Autodesk Inventor part; units mm, degrees
ref_plane "YZ Plane" through (0, 0, 0) normal (1, 0, 0) x (0, 1, 0)
ref_plane "XZ Plane" through (0, 0, 0) normal (0, 1, 0) x (-1, 0, 0)
ref_plane "XY Plane" through (0, 0, 0) normal (0, 0, 1) x (1, 0, 0)
sketch "スケッチ1" plane through (0, 0, 0) normal (0, 1, 0) x (-1, 0, 0)
  line L0 (0, -21.0065) -> (0, 21.0391)
  line L1 (-95.27, 0) -> (121.47, 0)
  line L2 (22, -15) -> (-22, -15)
  line L3 (-22, -15) -> (-22, 15)
  line L4 (-22, 15) -> (22, 15)
  line L5 (22, 15) -> (22, -15)
  line L6 (6, 15) -> (2.9, 15)
  line L7 (2.9, 15) -> (2.9, 11.5)
  line L8 (2.9, 11.5) -> (6, 11.5)
  line L9 (6, 11.5) -> (6, 15)
  arc A0 (10.85, 15) -> (9.45, 0) centre (90.5071, 0) ccw
  arc A1 (16.75, 0) -> (15.35, 15) centre (-64.3071, 0) ccw
  line L10 (13.1, -2.0457) -> (13.1, 1.915)
  line L11 (16.75, 0) -> (9.45, 0)
  line L12 (15.35, 15) -> (10.85, 15)
  line L13 (16.5956, 5) -> (9.6044, 5)
  line L14 (19.25, -15) -> (19.25, 15)
  point P0 (0, 0)
  point P1 (2.9, 15)
  point P2 (19.25, 0)
  point P3 (22, 0)
  dimension "d0" = 44
  dimension "d1" = 30
  dimension "d18" = 3.5
  dimension "d19" = 6
  dimension "d20" = 3.1
  dimension "d21" = 16.75
  dimension "d22" = 7.3
  dimension "d25" = 4.5
  dimension "d26" = 10
  dimension "d28" = 6.9913
  dimension "d37" = 2.9
  dimension "d38" = 19.25
extrude "押し出し1" add sketch "スケッチ1" against normal blind 2
extrude "押し出し3" add sketch "スケッチ1" along normal blind 3 contours L4 L9 L8 L7 | A0 L4 A1 L13
extrude "押し出し4" add sketch "スケッチ1" along normal blind 1.5 contours A0 L13 A1 L1
mirror "ミラー1" about plane through (0, 0, 0) normal (0, 0, 1) of "押し出し1", "押し出し3", "押し出し4"
extrude "押し出し5" add sketch "スケッチ1" along normal blind 4.2 contours L14 L1 L5 L2 | L14 L4 L5 L1
mirror "ミラー3" about plane through (0, 0, 0) normal (1, 0, 0) of "押し出し1", "押し出し3", "押し出し4", "ミラー1", "押し出し5"
sketch "スケッチ2" plane through (0, 0, 0) normal (0, 0, 1) x (1, 0, 0)
  line L0 (0, 5.44) -> (0, -3.24)
  line L1 (-30.8, 0) -> (30.8, 0)
  line L2 (-29.5, 14.3) -> (-27.5, 14.3)
  line L3 (-27.5, 14.3) -> (-27.5, 0)
  line L4 (27.5, 0) -> (27.5, 14.3)
  line L5 (27.5, 14.3) -> (29.5, 14.3)
  line L6 (29.5, 14.3) -> (29.5, -1.4)
  line L7 (29.5, -1.4) -> (25, -5.9)
  line L8 (25, -5.9) -> (-25, -5.9)
  line L9 (-25, -5.9) -> (-29.5, -1.4)
  line L10 (-29.5, -1.4) -> (-29.5, 14.3)
  line L11 (-19.25, 4.2) -> (-22, 4.2)
  line L12 (19.25, 4.2) -> (22, 4.2)
  line L13 (-22, -2) -> (-22, 4.2)
  line L14 (-22, 0) -> (-22, 4.2)
  line L15 (-22, 4.2) -> (-24.4249, 0)
  line L16 (22, -2) -> (22, 4.2)
  line L17 (22, 0) -> (22, 4.2)
  line L18 (22, 4.2) -> (24.4249, 0)
  line L19 (-27.5, 0) -> (-24.4249, 0)
  line L20 (-22, 0) -> (22, 0)
  line L21 (24.4249, 0) -> (27.5, 0)
  point P0 (0, 0)
  point P1 (24.4249, 0)
  point P2 (22, 0)
  point P3 (-22, 0)
  point P4 (-24.4249, 0)
  dimension "d41" = 59
  dimension "d42" = 2
  dimension "d44" = 20.2
  dimension "d45" = 45
  dimension "d46" = 50
  dimension "d47" = 120
  dimension "d50" = 14.3
extrude "押し出し6" add sketch "スケッチ2" along normal mid plane 30
chamfer "面取り1" distance 0.4 angle 45 22 edges at (-29.5, 6.45, 15) (-28.5, 14.3, 15) (-27.5, 7.15, 15) (-27.25, -3.65, 15) (0, -5.9, 15) (27.25, -3.65, 15) (29.5, 6.45, 15) (28.5, 14.3, 15) (27.5, 7.15, 15) (-29.5, 6.45, -15) (-28.5, 14.3, -15) (-27.5, 7.15, -15) (-27.25, -3.65, -15) (0, -5.9, -15) (27.25, -3.65, -15) (29.5, 6.45, -15) (28.5, 14.3, -15) (27.5, 7.15, -15) (-29.5, 14.3, 0) (-27.5, 14.3, 0) (27.5, 14.3, 0) (29.5, 14.3, 0)
equation "\"d39\" = 0.5 * RailHeight"
properties part number "PillarTopVD"
Source: CAD feature listing. Evaluate the final solid. Frame: model axes, mm. A direction names the side the tool comes from. Round coordinates to 2 decimals unless told otherwise and drop trailing zeros. Loops run counter-clockwise (first coordinate to the right, second up) from the corner with the lowest first, then second, coordinate; pieces in that order, holes last. Notation, with made-up numbers: M 82.25,-2.5 L 87.25,-2.5 A33 cw 87.25,32.5 Z; hole C 44.25,58 d5. An arc over 180 degrees is marked long. Use a Markdown table: item, result. Add a question column.
1. Section query A-A on y = 9.5. Return the cut outline in (x, z), then the cut area to 3 significant figures.
2. Line query: line 1 (Z direction, x = -11, y = 2.5); line 2 (X direction, y = 12.75, z = -2); line 3 (Y direction, x = 0.5, z = -12). Output: solid intervals per line, ascending.
3. Section query B-B on x = -12.5. Return the cut outline in (y, z), then the cut area to 3 significant figures.
4. Mould query, pull axis Z, two halves, no side actions, for faces 4 (the flat face through (13, 2, 5)), 5 (the flat face through (27.14, -3.48, -14.8)), 6 (the flat face through (-13, 3, -10)). Classes: pulls with the +Z half, pulls with the -Z half, needs draft (parallel to the pull), parting line crosses it, or undercut.
5. Contact query for flat-ended pins moving along their axis: P1, Ø8, axis at x = -11.5, z = 2.5, coming from the +Y side; P2, Ø1.2, axis at x = 18, z = 6, coming from the +Y side; P3, Ø1.4, axis at x = 20.5, z = 0.5, coming from the +Y side. Output: stop coordinate, or through.
6. Section query D-D on y = -2.75. Return the cut outline in (x, z), then the cut area to 3 significant figures.
7. Reachability of faces 1 (the flat face through (4, 1, 11.5)), 2 (the flat face through (-27.2, -3.7, -0.2)), 3 (the flat face through (-2.9, 1, -13)) from +Z, -Z, +X, -X, +Y, -Y: full face, straight path, thin tool, end or side. Return the list, or none.
Reported:
| question | item | result |
|---|---|---|
| 1 | outline | M -29.5,-14.6 L -29.1,-15 L -27.9,-15 L -27.5,-14.6 L -27.5,14.6 L -27.9,15 L -29.1,15 L -29.5,14.6 Z; M 27.5,-14.6 L 27.9,-15 L 29.1,-15 L 29.5,-14.6 L 29.5,14.6 L 29.1,15 L 27.9,15 L 27.5,14.6 Z |
| 1 | area | 119 mm² |
| 2 | line 1 | z = -15 to -5, 5 to 15 |
| 2 | line 2 | x = -29.5 to -27.5, 27.5 to 29.5 |
| 2 | line 3 | y = -5.9 to 0 |
| 3 | outline | M -5.9,-14.6 L -5.5,-15 L 3,-15 L 3,-5 L 1.5,-5 L 1.5,5 L 3,5 L 3,15 L -5.5,15 L -5.9,14.6 Z |
| 3 | area | 252 mm² |
| 4 | face 4 | undercut |
| 4 | face 5 | pulls with the -Z half |
| 4 | face 6 | needs draft |
| 5 | P1 | stops at y = 3 |
| 5 | P2 | stops at y = 0 |
| 5 | P3 | stops at y = 4.2 |
| 6 | outline | M -28.15,-14.6 L -27.58,-15 L 27.58,-15 L 28.15,-14.6 L 28.15,14.6 L 27.58,15 L -27.58,15 L -28.15,14.6 Z |
| 6 | area | 1,690 mm² |
| 7 | face 1 | +Y |
| 7 | face 2 | +Z, -Z, -X, -Y |
| 7 | face 3 | +Z, -Z, +Y |
